from build123d import *

# Parameters (mm, degrees)
SKETCH1_W           = 80
SKETCH1_H           = 50
BOSS_EXTRUDE1_DEPTH = 50
CUT_EXTRUDE1_DEPTH  = 10
CUT_EXTRUDE2_DEPTH  = 56
SKETCH4_W           = 30
SKETCH4_H           = 10
CUT_EXTRUDE3_DEPTH  = 56
SKETCH5_W           = 82.14120513
SKETCH5_H           = 20
CUT_EXTRUDE4_DEPTH  = 20


with BuildPart() as part:
    # Sketch1 → Boss-Extrude1 (new body)
    with BuildSketch(Plane.XY):
        with Locations((40, 25)):
            Rectangle(SKETCH1_W, SKETCH1_H)
    extrude(amount=-BOSS_EXTRUDE1_DEPTH)

    # Sketch2 → Cut-Extrude1 (cut)
    with BuildSketch(Plane.XY):
        Polygon((0, 30), (0, 50), (80, 50), (80, 0), (30, 0), (10, 30), align=None)
    extrude(amount=-CUT_EXTRUDE1_DEPTH, mode=Mode.SUBTRACT)

    # Sketch3 → Cut-Extrude2 (cut)
    with BuildSketch(Plane.XY.offset(-10)):
        Polygon((50, 50), (80, 20), (80, 50), align=None)
    extrude(amount=-CUT_EXTRUDE2_DEPTH, mode=Mode.SUBTRACT)

    # Sketch4 → Cut-Extrude3 (cut)
    with BuildSketch(Plane.XZ):
        with Locations((65, -15)):
            Rectangle(SKETCH4_W, SKETCH4_H)
    extrude(amount=-CUT_EXTRUDE3_DEPTH, mode=Mode.SUBTRACT)

    # Sketch5 → Cut-Extrude4 (cut)
    with BuildSketch(Plane(origin=(0, 50, 0), x_dir=(1, 0, 0), z_dir=(0, 1, 0))):
        with Locations((71.070602565, 20)):
            Rectangle(SKETCH5_W, SKETCH5_H)
    extrude(amount=-CUT_EXTRUDE4_DEPTH, mode=Mode.SUBTRACT)


solid = part.part
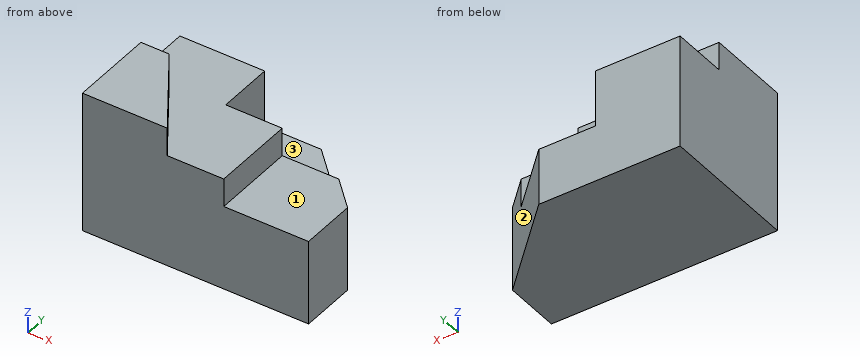
Read the model definition and answer for the solid it produces. Units are mm, in the model's axes. Face numbers are marked on the shaded views. A direction names the side the tool comes from. Round coordinates to 2 decimals unless told otherwise and drop trailing zeros. Write each loop counter-clockwise with the first axis right and the second up, starting at its lowest first coordinate (ties: lowest second). Pieces come first, ordered by that corner, then holes. Notation, with made-up numbers: (47, 16) - (67, 16) arc R18 cw to (67, 23) - close; hole circle Ø5 at (84, 59). An arc over 180 degrees is marked (long way). One line per question, with ' | ' between items. Start each with the question number.
1. Section D-D (y = 36.5) is taken. Determine the outline of the cut face in (x, z), and give its area (3 significant figures).
2. For the marked faces 1, 2 and 3, determine the directions among +Z, -Z, +X, -X, +Y, -Y from which every point of the face is accessible in a straight line to the end or side of a thin tool.
3. Section B-B (x = 14) is taken. Determine the outline of the cut face in (y, z).
4. Section A-A (y = 15) is taken. Determine the outline of the cut face in (x, z).
5. Section C-C (z = -43) is taken. Determine the outline of the cut face in (x, y).
6. Each of these flat-tipped pins is pushed along its axis until it touches: pin 1 (15 mm diameter, centred on x = 19, y = 19, fed in from +Z); pin 2 (5 mm diameter, centred on x = 45.5, z = -25, fed in from +Y); pin 3 (1.5 mm diameter, centred on x = 49.5, y = 16, fed in from +Z); pin 4 (24 mm diameter, centred on x = 63, y = 15, fed in from +Z). Where does it stop, or does it pass through?
7. Find the intervals of material crossed by probe 1 along Z at (x, y) = (49.5, 29); probe 2 along Z at (x, y) = (72, 15); probe 3 along Y at (x, z) = (38.5, -13), in increasing order. Write a range as [from, to].
Filled in:
1) outline: (0, -50) - (63.5, -50) - (63.5, -30) - (30, -30) - (30, -10) - (0, -10) - close | area: 1,870 mm²
2) face 1: +Z, +X, +Y, -Y | face 2: +Z, -Z, +X, +Y | face 3: +Z, +X, +Y
3) outline: (0, -50) - (50, -50) - (50, -10) - (24, -10) - (24, 0) - (0, 0) - close
4) outline: (0, -50) - (80, -50) - (80, -20) - (50, -20) - (50, -10) - (20, -10) - (20, 0) - (0, 0) - close
5) outline: (0, 0) - (80, 0) - (80, 20) - (50, 50) - (0, 50) - close
6) pin 1: z = 0 | pin 2: y = 30 | pin 3: z = -10 | pin 4: z = -20
7) probe 1: [-50, -10] | probe 2: [-50, -20] | probe 3: [0, 30]
